Read the model definition and answer for the solid it produces. Units are mm, in the model's axes. Face numbers are marked on the shaded views. A direction names the side the tool comes from. Coordinates: 2 decimals unless noted, no trailing zeros. Order: outer loops, then holes, each group sorted by start corner. A loop starts at its lowest first (then second) coordinate and runs counter-clockwise, first axis right, second up. Notation, with made-up numbers: (-24, 8) -> (31, 8) arc R9 ccw to (31, 12) -> close; hole circle Ø2 at (13, -15.5). An arc over 180 degrees is marked (long way). Answer in a Markdown table with one row per item.
Autodesk Inventor part; units mm, degrees
ref_plane "YZ Plane" through (0, 0, 0) normal (1, 0, 0) x (0, 1, 0)
ref_plane "XZ Plane" through (0, 0, 0) normal (0, 1, 0) x (-1, 0, 0)
ref_plane "XY Plane" through (0, 0, 0) normal (0, 0, 1) x (1, 0, 0)
sketch "スケッチ1" plane through (0, 0, 0) normal (1, 0, 0) x (0, 1, 0)
  circle A0 centre (0, 0) radius 19.05
  dimension "d0" = 38.1
extrude "押し出し1" add sketch "スケッチ1" along normal blind 22
hole "穴1" at (22, 0, 0) direction (-1, 0, 0) diameter 5.2 end through all
sketch "スケッチ2" plane through (22, 0, 0) normal (1, 0, 0) x (0, 0, -1)
  circle A0 centre (0, 0) radius 5.5
  dimension "d12" = 11
extrude "押し出し2" add sketch "スケッチ2" along normal blind 0.7
sketch "スケッチ3" plane through (0, 0, 0) normal (-1, 0, 0) x (0, 0, 1)
  circle A0 centre (0, 0) radius 5.5
  dimension "d15" = 11
extrude "押し出し3" add sketch "スケッチ3" along normal blind 0.7
fillet "フィレット1" radius 5 1 edges at (0, -19.05, 0)
fillet "フィレット2" radius 5 1 edges at (22, -19.05, 0)
sketch "スケッチ4" plane through (-0.7, 0, 0) normal (-1, 0, 0) x (0, 0, 1)
  line L0 (-2.3094, -4) -> (-4.6188, 0)
  line L1 (-4.6188, 0) -> (-2.3094, 4)
  line L2 (-2.3094, 4) -> (2.3094, 4)
  line L3 (2.3094, 4) -> (4.6188, 0)
  line L4 (4.6188, 0) -> (2.3094, -4)
  line L5 (2.3094, -4) -> (-2.3094, -4)
  point P0 (0, 0)
  point P1 (0, 0)
  point P2 (0, -4)
sketch "スケッチ5" plane through (22.7, 0, 0) normal (1, 0, 0) x (0, 0, -1)
  line L0 (2.3094, 4) -> (4.6188, 0)
  line L1 (4.6188, 0) -> (2.3094, -4)
  line L2 (2.3094, -4) -> (-2.3094, -4)
  line L3 (-2.3094, -4) -> (-4.6188, 0)
  line L4 (-4.6188, 0) -> (-2.3094, 4)
  line L5 (-2.3094, 4) -> (2.3094, 4)
  point P0 (0, 0)
  point P1 (0, 0)
  point P2 (0, 4)
extrude "押し出し4" cut sketch "スケッチ4" against normal blind 10
extrude "押し出し5" cut sketch "スケッチ5" against normal blind 10
properties part number "38omuni14184"
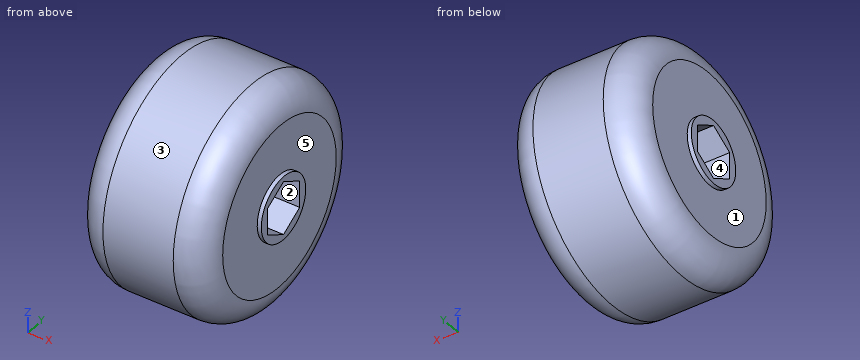
Q1. For a pull along Z with two mould halves and no side action, classify the marked faces 3, 4 and 5 as pulls with the +Z half, pulls with the -Z half, needs draft (parallel to the pull), parting line crosses it, or undercut.
Outcome:
| item | result |
|---|---|
| face 3 | parting line crosses it |
| face 4 | undercut |
| face 5 | needs draft |
Q2. For the marked faces 1 and 2, determine the directions among +Z, -Z, +X, -X, +Y, -Y from which every point of the face is accessible in a straight line to the end or side of a thin tool.
Outcome:
| item | result |
|---|---|
| face 1 | -X |
| face 2 | +X |
Q3. The part is cut by section A-A (z = 0). Write down the section's boundary in (x, y).
Outcome:
| item | result |
|---|---|
| outline | (-0.7, -5.5) -> (0, -5.5) -> (0, -14.05) arc R5 ccw to (5, -19.05) -> (17, -19.05) arc R5 ccw to (22, -14.05) -> (22, -5.5) -> (22.7, -5.5) -> (22.7, -4) -> (12.7, -4) -> (12.7, -2.6) -> (9.3, -2.6) -> (9.3, -4) -> (-0.7, -4) -> close; (-0.7, 4) -> (9.3, 4) -> (9.3, 2.6) -> (12.7, 2.6) -> (12.7, 4) -> (22.7, 4) -> (22.7, 5.5) -> (22, 5.5) -> (22, 14.05) arc R5 ccw to (17, 19.05) -> (5, 19.05) arc R5 ccw to (0, 14.05) -> (0, 5.5) -> (-0.7, 5.5) -> close |
Q4. The part is cut by section C-C (x = 3.5). Write down the section's boundary in (y, z), then the cut area to 3 significant figures.
Outcome:
| item | result |
|---|---|
| outline | circle Ø37.64 at (0, 0); hole (-4, -2.31) -> (0, -4.62) -> (4, -2.31) -> (4, 2.31) -> (0, 4.62) -> (-4, 2.31) -> close |
| area | 1,060 mm² |
Q5. Consider line 1 (Z direction, x = 11.1, y = 0); line 2 (X direction, y = -9.5, z = 9); line 3 (Y direction, x = 5.25, z = -4.5). Determine where each line is inside the solid, lowest interval first.
Outcome:
| item | result |
|---|---|
| line 1 | -19.05 to -2.6, 2.6 to 19.05 |
| line 2 | 0 to 22 |
| line 3 | -18.51 to -0.21, 0.21 to 18.51 |
Q6. Given pin 1 (3 mm diameter, centred on x = 4, z = -8, fed in from -Y); pin 2 (10 mm diameter, centred on y = -0.5, z = -15, fed in from +X); pin 3 (8 mm diameter, centred on x = 10, z = -13, fed in from -Y); pin 4 (4 mm diameter, centred on y = 0, z = 0, fed in from -X), each flat-ended and moving along its own axis, determine where each tip first touches the part or whether it passes through.
Outcome:
| item | result |
|---|---|
| pin 1 | y = -17.85 |
| pin 2 | x = 22 |
| pin 3 | y = -16.79 |
| pin 4 | through |
Q7. The part is cut by section B-B (x = 13.75). Write down the section's boundary in (y, z), then the cut area to 3 significant figures.
Outcome:
| item | result |
|---|---|
| outline | circle Ø38.1 at (0, 0); hole (-4, -2.31) -> (0, -4.62) -> (4, -2.31) -> (4, 2.31) -> (0, 4.62) -> (-4, 2.31) -> close |
| area | 1,080 mm² |
